Input: part model. Units: mm. Frame: model coordinates. A direction names the side the tool comes from. Round coordinates to 2 decimals unless told otherwise and drop trailing zeros. Order: outer loops, then holes, each group sorted by start corner. A loop starts at its lowest first (then second) coordinate and runs counter-clockwise, first axis right, second up. Notation, with made-up numbers: (47.5, 81.5) -> (95.5, 81.5) arc R22 cw to (95.5, 112.5) -> close; hole circle Ø1 at (40, 28.25). An arc over 180 degrees is marked (long way). Use a Markdown table: item, result.
from build123d import *

# Parameters (mm, degrees)
SKETCH1_W           = 170
SKETCH1_H           = 110
BOSS_EXTRUDE1_DEPTH = 88
FILLET1_R           = 10
SHELL1_START        = -75
SHELL1_OUTLINE_W    = 90
SHELL1_OUTLINE_H    = 72
SHELL1_DEPTH        = 150
SKETCH2_R           = 22.5
CUT_EXTRUDE1_DEPTH  = 135.141716107
SKETCH3_R           = 27.6
CUT_EXTRUDE2_DEPTH  = 13
FILLET2_R           = 8
SKETCH5_R           = 13.1
CUT_EXTRUDE3_DEPTH  = 8
SKETCH6_R           = 10.1
CUT_EXTRUDE4_DEPTH  = 0.8
CHAMFER1_SIZE       = 0.8
FILLET3_R           = 1
SKETCH7_W           = 35
SKETCH7_H           = 80
BOSS_EXTRUDE2_DEPTH = 10
FILLET5_R           = 10
CHAMFER2_SIZE       = 2
SKETCH8_R           = 4
CUT_EXTRUDE5_DEPTH  = 173.754160587
CHAMFER3_SIZE       = 0.5
SKETCH9_R           = 3.2
CUT_EXTRUDE6_DEPTH  = 12
SKETCH10_R          = 3.25
CUT_EXTRUDE7_DEPTH  = 12
CHAMFER4_SIZE       = 0.6
SKETCH11_R          = 10
CUT_EXTRUDE8_DEPTH  = 143.509648796
SKETCH12_R          = 10
CUT_EXTRUDE9_DEPTH  = 221.893639564
SKETCH13_R          = 10
CUT_EXTRUDE12_DEPTH = 179.728844902


# Read off the part's stored shape, not the designer's step: Shell1
# Some blends are built 0.0001 mm under size
with BuildPart() as part:
    # Sketch1 → Boss-Extrude1 (new body)
    with BuildSketch(Plane.XY):
        Rectangle(SKETCH1_W, SKETCH1_H)
    extrude(amount=BOSS_EXTRUDE1_DEPTH)

    # Fillet1
    fillet1_edges = [part.edges().sort_by_distance(p)[0] for p in [
        (85, -55, 44),
        (-85, -55, 44),
        (-85, 55, 44),
        (85, 55, 44),
    ]]
    fillet(fillet1_edges, radius=FILLET1_R)

    # Shell1 outline → Shell1 (cut)
    with BuildSketch(Plane.YZ.offset(SHELL1_START)):
        with Locations((0, 36)):
            Rectangle(SHELL1_OUTLINE_W, SHELL1_OUTLINE_H)
    extrude(amount=SHELL1_DEPTH, mode=Mode.SUBTRACT)

    # Sketch2 → Cut-Extrude1 (cut, through all)
    with BuildSketch(Plane.XY.offset(88)):
        Circle(SKETCH2_R)
    extrude(amount=-CUT_EXTRUDE1_DEPTH, mode=Mode.SUBTRACT)

    # Sketch3 → Cut-Extrude2 (cut)
    with BuildSketch(Plane(origin=(0, 0, 72), x_dir=(-1, 0, 0), z_dir=(0, 0, -1))):
        Circle(SKETCH3_R)
    extrude(amount=-CUT_EXTRUDE2_DEPTH, mode=Mode.SUBTRACT)

    # Fillet2
    fillet2_edges = [part.edges().sort_by_distance(p)[0] for p in [
        (0, -55, 88),
        (-85, 0, 88),
        (85, 0, 88),
        (0, 55, 88),
        (-82.071067812, 52.071067812, 88),
        (82.071067812, 52.071067812, 88),
        (82.071067812, -52.071067812, 88),
        (-82.071067812, -52.071067812, 88),
    ]]
    fillet(fillet2_edges, radius=FILLET2_R)

    # Sketch5 → Cut-Extrude3 (cut)
    with BuildSketch(Plane(origin=(0, 0, 72), x_dir=(-1, 0, 0), z_dir=(0, 0, -1))):
        with Locations((-50, 0)):
            Circle(SKETCH5_R)
    extrude(amount=-CUT_EXTRUDE3_DEPTH, mode=Mode.SUBTRACT)

    # Sketch6 → Cut-Extrude4 (cut)
    with BuildSketch(Plane(origin=(0, 0, 80), x_dir=(-1, 0, 0), z_dir=(0, 0, -1))):
        with Locations((-50, 0)):
            Circle(SKETCH6_R)
    extrude(amount=-CUT_EXTRUDE4_DEPTH, mode=Mode.SUBTRACT)

    # Chamfer1
    chamfer1_edges = [part.edges().sort_by_distance(p)[0] for p in [
        (27.6, 0, 72),
        (-22.5, 0, 85),
        (63.1, 0, 72),
        (60.1, 0, 80),
    ]]
    chamfer(chamfer1_edges, length=CHAMFER1_SIZE - 0.0001)  # a hair under: the kernel refuses the full size

    # Fillet3
    fillet3_edges = [part.edges().sort_by_distance(p)[0] for p in [
        (-22.5, 0, 88),
    ]]
    fillet(fillet3_edges, radius=FILLET3_R)

    # Sketch7 → Boss-Extrude2 (add)
    with BuildSketch(Plane.XZ.offset(55)):
        with Locations((-92.5, 40)):
            Rectangle(SKETCH7_W, SKETCH7_H)
        with Locations((92.5, 40)):
            Rectangle(SKETCH7_W, SKETCH7_H)
    extrude(amount=-BOSS_EXTRUDE2_DEPTH)

    # Fillet5
    fillet5_edges = [part.edges().sort_by_distance(p)[0] for p in [
        (-110, -50, 80),
        (-110, -50, 0),
        (110, -50, 0),
        (110, -50, 80),
    ]]
    fillet(fillet5_edges, radius=FILLET5_R)

    # Chamfer2
    # the kernel refuses this chamfer: 2 mm, written as the material it takes off along each edge
    with BuildSketch(Plane(origin=(85, -45, 0), x_dir=(0, -0.9996219169112968, -0.02749587661058639), z_dir=(1, 0, 0)), Plane(origin=(-100, -45, 0), x_dir=(0, -0.9996219169112968, -0.02749587661058639), z_dir=(1, 0, 0))) as chamfer2_piece_1:
        Polygon((CHAMFER2_SIZE * 0.999621916911, -CHAMFER2_SIZE * 0.0274958766106), (-CHAMFER2_SIZE * 0.0274958766106, -CHAMFER2_SIZE * 0.999621916911), (0, 0), align=None)
    extrude(amount=15, mode=Mode.SUBTRACT)
    with BuildSketch(Plane(origin=(100, -45, 80), x_dir=(0, 0.02749587661058555, -0.9996219169112968), z_dir=(-1, 0, 0)), Plane(origin=(-85, -45, 80), x_dir=(0, 0.02749587661058555, -0.9996219169112968), z_dir=(-1, 0, 0))) as chamfer2_piece_2:
        Polygon((CHAMFER2_SIZE * 0.999621916911, CHAMFER2_SIZE * 0.0274958766106), (-CHAMFER2_SIZE * 0.0274958766106, CHAMFER2_SIZE * 0.999621916911), (0, 0), align=None)
    extrude(amount=15, mode=Mode.SUBTRACT)
    with BuildSketch(Plane(origin=(110, -45, 10), x_dir=(-0.9996219169112968, 0.02749587661058555, 0), z_dir=(0, 0, 1)), Plane(origin=(-110, -45, 70), x_dir=(0.9996219169112968, 0.02749587661058555, 0), z_dir=(0, 0, -1))) as chamfer2_piece_3:
        Polygon((CHAMFER2_SIZE * 0.999621916911, CHAMFER2_SIZE * 0.0274958766106), (-CHAMFER2_SIZE * 0.0274958766106, CHAMFER2_SIZE * 0.999621916911), (0, 0), align=None)
    extrude(amount=60, mode=Mode.SUBTRACT)
    with BuildSketch(Plane(origin=(100, -45, 70), x_dir=(1, 0, 0), z_dir=(0, 0, -1))) as chamfer2_piece_4:
        Polygon((10 - CHAMFER2_SIZE, 0), (10, CHAMFER2_SIZE), (10, 0), align=None)
    revolve(axis=Axis((100, -45, 70), (0, -1, 0)), revolution_arc=90, mode=Mode.SUBTRACT)
    with BuildSketch(Plane(origin=(100, -45, 10), x_dir=(0, 0, -1), z_dir=(-1, 0, 0))) as chamfer2_piece_5:
        Polygon((10, CHAMFER2_SIZE), (10 - CHAMFER2_SIZE, 0), (10, 0), align=None)
    revolve(axis=Axis((100, -45, 10), (0, -1, 0)), revolution_arc=90, mode=Mode.SUBTRACT)
    with BuildSketch(Plane(origin=(-100, -45, 70), x_dir=(0, 0, 1), z_dir=(1, 0, 0))) as chamfer2_piece_6:
        Polygon((10 - CHAMFER2_SIZE, 0), (10, CHAMFER2_SIZE), (10, 0), align=None)
    revolve(axis=Axis((-100, -45, 70), (0, -1, 0)), revolution_arc=90, mode=Mode.SUBTRACT)
    with BuildSketch(Plane(origin=(-100, -45, 10), x_dir=(0, 0, -1), z_dir=(1, 0, 0))) as chamfer2_piece_7:
        Polygon((10, -CHAMFER2_SIZE), (10 - CHAMFER2_SIZE, 0), (10, 0), align=None)
    revolve(axis=Axis((-100, -45, 10), (0, 1, 0)), revolution_arc=90, mode=Mode.SUBTRACT)

    # Sketch8 → Cut-Extrude5 (cut, through all)
    with BuildSketch(Plane(origin=(0, -45, 0), x_dir=(1, 0, 0), z_dir=(0, 1, 0))):
        with Locations(Location((-97, -40, 0), (0, 0, 270))):
            Circle(SKETCH8_R)
        with Locations(Location((-97, -15, 0), (0, 0, 270))):
            Circle(SKETCH8_R)
        with Locations(Location((-97, -65, 0), (0, 0, 270))):
            Circle(SKETCH8_R)
    cut_extrude5 = extrude(amount=-CUT_EXTRUDE5_DEPTH, mode=Mode.SUBTRACT)

    # Mirror4: Cut-Extrude5 across plane
    add(cut_extrude5.mirror(Plane(origin=(0, 0, 0), x_dir=(0, 0, 1), z_dir=(1, 0, 0))), mode=Mode.SUBTRACT)

    # Chamfer3
    chamfer3_edges = [part.edges().sort_by_distance(p)[0] for p in [
        (-97, -45, 61),
        (-97, -45, 11),
        (-97, -45, 36),
        (97, -45, 61),
        (97, -45, 11),
        (97, -45, 36),
    ]]
    chamfer(chamfer3_edges, length=CHAMFER3_SIZE)

    # Sketch9 → Cut-Extrude6 (cut)
    with BuildSketch(Plane(origin=(0, 0, 0), x_dir=(-1, 0, 0), z_dir=(0, 0, -1))):
        with Locations((0, 50)):
            Circle(SKETCH9_R)
        with Locations((-50, 50)):
            Circle(SKETCH9_R)
        with Locations(Location((50, 50, 0), (0, 0, 180))):
            Circle(SKETCH9_R)
    cut_extrude6 = extrude(amount=-CUT_EXTRUDE6_DEPTH, mode=Mode.SUBTRACT)

    # Mirror5: Cut-Extrude6 across plane
    add(cut_extrude6.mirror(Plane.ZX), mode=Mode.SUBTRACT)

    # Sketch10 → Cut-Extrude7 (cut)
    with BuildSketch(Plane(origin=(0, 0, 0), x_dir=(-1, 0, 0), z_dir=(0, 0, -1))):
        with Locations((-80, 0)):
            Circle(SKETCH10_R)
        with Locations((-80, 40)):
            Circle(SKETCH10_R)
        with Locations(Location((-80, -40, 0), (0, 0, 180))):
            Circle(SKETCH10_R)
    cut_extrude7 = extrude(amount=-CUT_EXTRUDE7_DEPTH, mode=Mode.SUBTRACT)

    # Mirror6: Cut-Extrude7 across plane
    add(cut_extrude7.mirror(Plane(origin=(0, 0, 0), x_dir=(0, 0, 1), z_dir=(1, 0, 0))), mode=Mode.SUBTRACT)

    # Chamfer4
    chamfer4_edges = [part.edges().sort_by_distance(p)[0] for p in [
        (-53.2, 50, 0),
        (53.2, 50, 0),
        (3.2, 50, 0),
        (-53.2, -50, 0),
        (53.2, -50, 0),
        (3.2, -50, 0),
        (76.75, -40, 0),
        (83.25, 40, 0),
        (83.25, 0, 0),
        (-76.75, -40, 0),
        (-83.25, 40, 0),
        (-83.25, 0, 0),
    ]]
    chamfer(chamfer4_edges, length=CHAMFER4_SIZE)

    # Sketch11 → Cut-Extrude8 (cut, through all)
    with BuildSketch(Plane(origin=(0, 0, 72), x_dir=(-1, 0, 0), z_dir=(0, 0, -1))):
        Circle(SKETCH11_R)
        with Locations((50, 0)):
            Circle(SKETCH11_R)
        with Locations((50, 30)):
            Circle(SKETCH11_R)
        with Locations((50, -30)):
            Circle(SKETCH11_R)
        with Locations(Location((-50, -30, 0), (0, 0, 180))):
            Circle(SKETCH11_R)
        with Locations(Location((-50, 30, 0), (0, 0, 180))):
            Circle(SKETCH11_R)
    extrude(amount=-CUT_EXTRUDE8_DEPTH, mode=Mode.SUBTRACT)

    # Sketch12 → Cut-Extrude9 (cut, through all)
    with BuildSketch(Plane.ZY.offset(85)):
        with Locations(Location((23, 0, 0), (0, 0, 270))):
            Circle(SKETCH12_R)
        with Locations(Location((23, 30, 0), (0, 0, 270))):
            Circle(SKETCH12_R)
        with Locations(Location((23, -30, 0), (0, 0, 270))):
            Circle(SKETCH12_R)
        with Locations(Location((57, -30, 0), (0, 0, 90))):
            Circle(SKETCH12_R)
        with Locations(Location((57, 0, 0), (0, 0, 90))):
            Circle(SKETCH12_R)
        with Locations(Location((57, 30, 0), (0, 0, 90))):
            Circle(SKETCH12_R)
    extrude(amount=-CUT_EXTRUDE9_DEPTH, mode=Mode.SUBTRACT)

    # Sketch13 → Cut-Extrude12 (cut, through all)
    with BuildSketch(Plane(origin=(0, 55, 0), x_dir=(1, 0, 0), z_dir=(0, 1, 0))):
        with Locations(Location((-50, -23, 0), (0, 0, 270))):
            Circle(SKETCH13_R)
        with Locations(Location((-50, -58, 0), (0, 0, 270))):
            Circle(SKETCH13_R)
        with Locations(Location((0, -23, 0), (0, 0, 270))):
            Circle(SKETCH13_R)
        with Locations(Location((0, -58, 0), (0, 0, 270))):
            Circle(SKETCH13_R)
        with Locations(Location((50, -23, 0), (0, 0, 270))):
            Circle(SKETCH13_R)
        with Locations(Location((50, -58, 0), (0, 0, 270))):
            Circle(SKETCH13_R)
    extrude(amount=-CUT_EXTRUDE12_DEPTH, mode=Mode.SUBTRACT)


solid = part.part
1) Cut plane A-A on z = 40. Return loops of the section in (x, y).
Results found:
| item | result |
|---|---|
| outline | (-110, -55) -> (-101, -55) -> (-101, -45.5) -> (-101.5, -45) -> (-108, -45) -> (-110, -47) -> close; (-93, -55) -> (93, -55) -> (93, -45.5) -> (92.5, -45) -> (85, -45) -> (85, 45) arc R10 ccw to (75, 55) -> (-75, 55) arc R10 ccw to (-85, 45) -> (-85, -45) -> (-92.5, -45) -> (-93, -45.5) -> close; (101, -55) -> (110, -55) -> (110, -47) -> (108, -45) -> (101.5, -45) -> (101, -45.5) -> close; hole (-75, -45) -> (75, -45) -> (75, 45) -> (-75, 45) -> close |
2) Cut plane C-C on z = 23. Count the separate pieces of the cut face and the enclosed holes in it, and give its area (3 significant figures).
Results found:
| item | result |
|---|---|
| separate pieces | 12 |
| enclosed holes | 0 |
| area | 3,250 mm² |
3) Pin query (flat end, axial travel): pin 1 Ø23 at (y, z) = (0, 23) entering from +X; pin 2 Ø2 at (x, y) = (80, 1) entering from -Z; pin 3 Ø1.5 at (y, z) = (7.5, 24) entering from -X; pin 4 Ø5 at (x, y) = (-92.5, -47.5) entering from +Z. Return the tip coordinate at first contact, or that it passes through.
Results found:
| item | result |
|---|---|
| pin 1 | stops at x = 85 |
| pin 2 | stops at z = 12 |
| pin 3 | passes through |
| pin 4 | stops at z = 80 |
4) Cut plane B-B on x = -35. Return loops of the section in (y, z).
Results found:
| item | result |
|---|---|
| outline | (-55, 0) -> (-45, 0) -> (-45, 72) -> (45, 72) -> (45, 0) -> (55, 0) -> (55, 80) arc R8 ccw to (47, 88) -> (-47, 88) arc R8 ccw to (-55, 80) -> close |
5) Pull-direction query (X, two-part tool) for faces 1 (the cylindrical face through (-1.05, 52.594, 85.719)), 2 (the cylindrical face through (-107.15, -50.94, 3.01)), 3 (the cylindrical face through (41.128, 50.07, 27.614)), 4 (the cylindrical face through (82.15, 51.99, 40.56)); classes: +X half, -X half, draft (parallel to the pull), parting line (faces both ways), or undercut.
Results found:
| item | result |
|---|---|
| face 1 | draft |
| face 2 | -X half |
| face 3 | undercut |
| face 4 | +X half |
6) Line query: L1, parallel to Y at x = 0, z = 5.25; L2, parallel to Z at x = 97, y = -51.5; L3, parallel to X at y = -51.25, z = 58. Output: solid intervals per line, ascending. Write a range as [from, to].
Results found:
| item | result |
|---|---|
| L1 | y = [-55, -53.2], [-46.8, -45], [45, 46.8], [53.2, 55] |
| L2 | z = [0, 11], [19, 36], [44, 61], [69, 80] |
| L3 | x = [-110, -60], [-40, -10], [10, 40], [60, 110] |
7) Set-up query: faces 5 (the conical face through (106.13, -45.57, 75.99)), 6 (the flat face through (-80, 40, 12)). Return all of +Z, -Z, +X, -X, +Y, -Y with unobstructed straight access to the full face (end or side cutting, diameter ignored); none if empty.
Results found:
| item | result |
|---|---|
| face 5 | +Z, +X, +Y |
| face 6 | -Z |
